```python
from build123d import *

# Parameters (mm, degrees)
PARTS_W           = 29.2
PARTS_H           = 21.15
MAIN_FACE_DEPTH   = 2
SKETCH3_R         = 2.525
IR_CUT_DEPTH      = 2
TSOP_GROOVE_DEPTH = 1.5
SKETCH4_W         = 5.4
SKETCH4_H         = 3.4
TOF_CUT_DEPTH     = 2
SKETCH6_R         = 1.575
SHAFTS_DEPTH      = 5
CHAMFER1_SIZE     = 0.2
SKETCH7_W         = 15
SKETCH7_H         = 3.5
PINSLOTS_DEPTH    = 1
TOFWINDOW_SIZE    = 1


with BuildPart() as part:
    # Parts → Main Face (new body)
    with BuildSketch(Plane(origin=(0, 0, 0), x_dir=(1, 0, 0), z_dir=(0, 1, 0))):
        with Locations((0, 3.175)):
            Rectangle(PARTS_W, PARTS_H)
    extrude(amount=-MAIN_FACE_DEPTH)

    # Sketch3 → IR Cut (cut)
    with BuildSketch(Plane(origin=(0, 0, 0), x_dir=(1, 0, 0), z_dir=(0, 1, 0))):
        with Locations(Location((7.3875, 9.075, 0), (0, 0, 270))):
            Circle(SKETCH3_R)
        Polygon((-2.6125, 11.75), (-2.6125, 6.4), (-9.4125, 6.4), (-9.4125, 5.9), (-9.9125, 5.9), (-9.9125, 6.4), (-9.9125, 11.75), (-9.9125, 12.25), (-9.4125, 12.25), (-9.4125, 11.75), align=None)
    extrude(amount=-IR_CUT_DEPTH, mode=Mode.SUBTRACT)

    # Sketch5 → TSOP Groove (cut)
    with BuildSketch(Plane.XZ.offset(2)):
        Polygon((-2.6125, -11.75), (-2.6125, -6.4), (-2.6125, -5.9), (1.3875, -5.9), (1.3875, -6.4), (1.3875, -11.75), (1.3875, -12.25), (-2.6125, -12.25), align=None)
    extrude(amount=-TSOP_GROOVE_DEPTH, mode=Mode.SUBTRACT)

    # Sketch4 → TOF Cut (cut)
    with BuildSketch(Plane(origin=(0, 0, 0), x_dir=(1, 0, 0), z_dir=(0, 1, 0))):
        with Locations((0, 1.6)):
            Rectangle(SKETCH4_W, SKETCH4_H)
    extrude(amount=-TOF_CUT_DEPTH, mode=Mode.SUBTRACT)

    # Sketch6 → Shafts (add)
    with BuildSketch(Plane.XZ.offset(2)):
        with Locations(Location((-9.9, 0, 0), (0, 0, 270))):
            Circle(SKETCH6_R)
        with Locations(Location((9.9, 0, 0), (0, 0, 270))):
            Circle(SKETCH6_R)
    extrude(amount=SHAFTS_DEPTH)

    # Chamfer1
    chamfer1_edges = [part.edges().sort_by_distance(p)[0] for p in [
        (9.9, -7, 1.575),
        (-9.9, -7, 1.575),
    ]]
    chamfer(chamfer1_edges, length=CHAMFER1_SIZE)

    # Sketch7 → PinSlots (cut)
    with BuildSketch(Plane.XZ.offset(2)):
        with Locations((0, 3.15)):
            Rectangle(SKETCH7_W, SKETCH7_H)
    extrude(amount=-PINSLOTS_DEPTH, mode=Mode.SUBTRACT)

    # ToFWindow
    tofwindow_edges = [part.edges().sort_by_distance(p)[0] for p in [
        (-2.7, 0, -1.6),
        (0, 0, 0.1),
        (2.7, 0, -1.6),
        (0, 0, -3.3),
    ]]
    chamfer(tofwindow_edges, length=TOFWINDOW_SIZE)


solid = part.part
```
Read the model definition and answer for the solid it produces. Units are mm, in the model's axes. A direction names the side the tool comes from. Coordinates: 2 decimals unless noted, no trailing zeros. Write each loop counter-clockwise with the first axis right and the second up, starting at its lowest first coordinate (ties: lowest second). Pieces come first, ordered by that corner, then holes. Notation, with made-up numbers: (-12, -6.5) -> (41, -6.5) arc R18 ccw to (41, -1.5) -> close; hole circle Ø8 at (-12, -36.5). An arc over 180 degrees is marked (long way). Answer as a JSON object with one key per item and string values.
Q1. The part is cut by section B-B on z = -9. Give the vertices of the cut face in (x, y), then the cut area to 3 significant figures.
The answers:
{"outline": "(-14.6, -2) -> (-9.91, -2) -> (-9.91, 0) -> (-14.6, 0) -> close; (-2.61, -0.5) -> (1.39, -0.5) -> (1.39, -2) -> (4.86, -2) -> (4.86, 0) -> (-2.61, 0) -> close; (9.91, -2) -> (14.6, -2) -> (14.6, 0) -> (9.91, 0) -> close", "area": "27.7 mm2"}
Q2. The part is cut by section A-A on x = -3.25. Give the vertices of the cut face in (y, z).
The answers:
{"outline": "(-2, -13.75) -> (0, -13.75) -> (0, -11.75) -> (-2, -11.75) -> close; (-2, -6.4) -> (0, -6.4) -> (0, -4.3) -> (-0.45, -3.85) -> (-0.45, 0.65) -> (0, 1.1) -> (0, 7.4) -> (-2, 7.4) -> (-2, 4.9) -> (-1, 4.9) -> (-1, 1.4) -> (-2, 1.4) -> close"}
Q3. The part is cut by section C-C on y = -4.25. Give the vertices of the cut face in (x, z) (3 decimals), then the cut area to 3 significant figures.
The answers:
{"outline": "circle Ø3.15 at (-9.9, 0); circle Ø3.15 at (9.9, 0)", "area": "15.6 mm2"}
Q4. Determine the mould class of faces 1 (the cylindrical face through (-8.34, -4.37, 0.21)), 2 (the flat face through (-9.912, -1, -9)), 3 (the flat face through (-1, -1, -12.25)), 4 (the flat face through (-14.6, -1, -3)) for opening direction Z: pulls with the +Z half, pulls with the -Z half, needs draft (parallel to the pull), parting line crosses it, or undercut.
The answers:
{"face 1": "parting line crosses it", "face 2": "undercut", "face 3": "undercut", "face 4": "needs draft"}
Q5. A flat-ended cylindrical pin translates along its axis: pin 1 Ø4.5 at (x, z) = (0, -9.5) entering from -Y. Find the tip coordinate at first contact, or state that the pin passes through.
The answers:
{"pin 1": "stops at y = -2"}
Q6. The part is cut by section D-D on z = 3.5. Give the vertices of the cut face in (x, y), then the cut area to 3 significant figures.
The answers:
{"outline": "(-14.6, -2) -> (-7.5, -2) -> (-7.5, -1) -> (7.5, -1) -> (7.5, -2) -> (14.6, -2) -> (14.6, 0) -> (-14.6, 0) -> close", "area": "43.4 mm2"}
Q7. Consider line 1 (Z direction, x = -0.5, y = -0.75); line 2 (Y direction, x = -1, z = 2.25); line 3 (Y direction, x = 2, z = -8.75). Determine where each line is inside the solid, lowest interval first. Write a range as [from, to].
The answers:
{"line 1": "z = [-13.75, -12.25], [-5.9, -3.55], [0.35, 7.4]", "line 2": "y = [-1, 0]", "line 3": "y = [-2, 0]"}
Q8. A tool of negligible diameter and unlimited length cuts with its end or side. For faces 5 (the flat face through (-0.1, -0.5, 0.6)), 6 (the flat face through (-6, -1, -11.75)), 7 (the flat face through (-1, -1, -5.9)), from which of +Z, -Z, +X, -X, +Y, -Y can it reach the whole face along a straight path? Write none if from no direction.
The answers:
{"face 5": "+Y", "face 6": "+Y, -Y", "face 7": "-Y"}
